Part model, mm, in its own coordinate system. Round coordinates to 2 decimals unless told otherwise and drop trailing zeros. Order: outer loops, then holes, each group sorted by start corner. A loop starts at its lowest first (then second) coordinate and runs counter-clockwise, first axis right, second up. Notation, with made-up numbers: (-2, 43) -> (22, 43) arc R26 ccw to (22, 82) -> close; hole circle Ø9 at (88, 60). An arc over 180 degrees is marked (long way). Answer as a JSON object with one key per item and string values. Group by question number.
```python
from build123d import *

# Parameters (mm, degrees)
F5_R      = 76.2
F4_R      = 101.6
F7_R      = 76.2
F8_DEPTH  = 304.8
F9_R      = 75.7174
F12_DEPTH = 304.8
F10_R     = 75.7174
F11_R     = 101.1174


with BuildPart() as f6:
    # F5 (on face) → F6 section 0
    with BuildSketch(Plane(origin=(0, 0, 508), x_dir=(1, 0, 0), z_dir=(0, 0, -1))):
        Circle(F5_R)
    # F4 (on face) → F6 section 1
    with BuildSketch(Plane.XY):
        Circle(F4_R)
    loft()

    # F7 (on face) → F8 (join)
    with BuildSketch(Plane(origin=(327.647171, 0, 327.647171), x_dir=(0.707107, 0, -0.707107), z_dir=(0.707107, 0, 0.707107))):
        with Locations((-107.763073, 0)):
            Circle(F7_R)
    extrude(amount=-F8_DEPTH)

    # F9 (on face) → F12 (cut)
    with BuildSketch(Plane(origin=(327.647171, 0, 327.647171), x_dir=(0.707107, 0, -0.707107), z_dir=(0.707107, 0, 0.707107))):
        with Locations((-107.763073, 0)):
            Circle(F9_R)
    extrude(amount=-F12_DEPTH, mode=Mode.SUBTRACT)

    # F10 (on face) → F13 section 0
    with BuildSketch(Plane(origin=(0, 0, 508), x_dir=(1, 0, 0), z_dir=(0, 0, -1))):
        Circle(F10_R)
    # F11 (on face) → F13 section 1
    with BuildSketch(Plane.XY):
        Circle(F11_R)
    loft(mode=Mode.SUBTRACT)


solid = f6.part
```
Q1. Band-saw the part on B-B (z = 409.5). Count the separate pieces of the cut face and the enclosed holes in it, plus the area to 3 significant figures.
Q2. Band-saw the part on A-A (x = 0). List the corners of the cut face in (y, z).
Q3. Band-saw the part on D-D (z = 87). List the corners of the cut face in (x, y), plus the area to 3 significant figures.
Q4. Wall check: line 1 (Z direction, x = 108.5, y = -12); line 2 (Y direction, x = -83.5, z = 138); line 3 (Y direction, x = 94.5, z = 172). Give the ranges that are in metal, low to high. Write a range as [from, to].
Q5. Drop flat-ended pins along their axis: pin 1 Ø12 at (x, y) = (182.5, -17.5) entering from +Z; pin 2 Ø4 at (x, z) = (51.5, 176) entering from +Y; pin 3 Ø10 at (x, y) = (215, -14.5) entering from +Z. Give the stop position or say it passes through.
Completed:
{
 "1": {"separate pieces": "2", "enclosed holes": "1", "area": "397 mm2"},
 "2": {"outline": "(-101.6, 0) -> (-101.12, 0) -> (-75.72, 508) -> (-76.2, 508) -> close; (75.72, 508) -> (101.12, 0) -> (101.6, 0) -> (76.2, 508) -> close"},
 "3": {"outline": "circle Ø194.5 at (0, 0); hole circle Ø193.53 at (0, 0)", "area": "294 mm2"},
 "4": {"line 1": "[154.48, 155.17], [366.63, 367.32]", "line 2": "[-44.67, -43.64], [43.64, 44.67]", "line 3": "[-54.79, -54.11], [54.11, 54.79]"},
 "5": {"pin 1": "z = 446.08", "pin 2": "y = 78.5", "pin 3": "z = 267.51"}
}
